CAD build for the part. Positions are in the model's coordinates, mm. Face numbers are marked on the shaded views. A direction names the side the tool comes from. Give positions to 0.01 mm unless a question says otherwise; leave off trailing zeros. Loops run counter-clockwise (first coordinate to the right, second up) from the corner with the lowest first, then second, coordinate; pieces in that order, holes last. Notation, with made-up numbers: M -35.5,-12 L 5.5,-12 A15 cw 5.5,2 Z; hole C -2.5,-30 d3. An arc over 180 degrees is marked long. Answer as CSV lines item,"result".
from build123d import *

# Parameters (mm, degrees)
SKETCH1_W           = 10.5
SKETCH1_H           = 14
SKETCH1_R           = 0.75
SKETCH1_R_2         = 2.25
BOSS_EXTRUDE1_DEPTH = 1.3
SKETCH2_W           = 10.5
SKETCH2_H           = 1.5
BOSS_EXTRUDE2_DEPTH = 14
SKETCH3_W           = 1.4
SKETCH3_H           = 3.3
BOSS_EXTRUDE3_DEPTH = 15.3
SKETCH4_W           = 10.5
SKETCH4_H           = 0.5
BOSS_EXTRUDE4_DEPTH = 1.3
SKETCH5_W           = 10.5
SKETCH5_H           = 1.5
BOSS_EXTRUDE5_DEPTH = 10
SKETCH6_W           = 1
SKETCH6_H           = 13
BOSS_EXTRUDE6_DEPTH = 3
CHAMFER1_SIZE       = 1


with BuildPart() as part:
    # Sketch1 → Boss-Extrude1 (new body)
    with BuildSketch(Plane(origin=(0, 0, 0), x_dir=(1, 0, 0), z_dir=(0, 1, 0))):
        Rectangle(SKETCH1_W, SKETCH1_H)
        with Locations(Location((-3, 3, 0), (0, 0, 270))):
            Circle(SKETCH1_R, mode=Mode.SUBTRACT)
        with Locations(Location((3, 3, 0), (0, 0, 270))):
            Circle(SKETCH1_R, mode=Mode.SUBTRACT)
        with Locations(Location((-3, -3, 0), (0, 0, 270))):
            Circle(SKETCH1_R, mode=Mode.SUBTRACT)
        with Locations(Location((3, -3, 0), (0, 0, 270))):
            Circle(SKETCH1_R, mode=Mode.SUBTRACT)
        with Locations(Location((0, 0, 0), (0, 0, 270))):
            Circle(SKETCH1_R_2, mode=Mode.SUBTRACT)
    extrude(amount=BOSS_EXTRUDE1_DEPTH)

    # Sketch2 → Boss-Extrude2 (add)
    with BuildSketch(Plane(origin=(0, 1.3, 0), x_dir=(1, 0, 0), z_dir=(0, 1, 0))):
        with Locations((0, -6.25)):
            Rectangle(SKETCH2_W, SKETCH2_H)
    extrude(amount=BOSS_EXTRUDE2_DEPTH)

    # Sketch3 → Boss-Extrude3 (add)
    with BuildSketch(Plane.XZ):
        with Locations((-4.55, 8.65)):
            Rectangle(SKETCH3_W, SKETCH3_H)
        with Locations((4.55, 8.65)):
            Rectangle(SKETCH3_W, SKETCH3_H)
    extrude(amount=-BOSS_EXTRUDE3_DEPTH)

    # Sketch4 → Boss-Extrude4 (add)
    with BuildSketch(Plane.XZ):
        with Locations((0, -7.25)):
            Rectangle(SKETCH4_W, SKETCH4_H)
    extrude(amount=-BOSS_EXTRUDE4_DEPTH)

    # Sketch5 → Boss-Extrude5 (add)
    with BuildSketch(Plane.XZ):
        with Locations((0, -8.25)):
            Rectangle(SKETCH5_W, SKETCH5_H)
    extrude(amount=-BOSS_EXTRUDE5_DEPTH)

    # Sketch6 → Boss-Extrude6 (add)
    with BuildSketch(Plane(origin=(0, 1.3, 0), x_dir=(1, 0, 0), z_dir=(0, 1, 0))):
        with Locations((4.75, 1)):
            Rectangle(SKETCH6_W, SKETCH6_H)
        with Locations((-4.75, 1)):
            Rectangle(SKETCH6_W, SKETCH6_H)
    extrude(amount=BOSS_EXTRUDE6_DEPTH)

    # Chamfer1
    chamfer1_edges = [part.edges().sort_by_distance(p)[0] for p in [
        (0, 1.3, -7.5),
    ]]
    chamfer(chamfer1_edges, length=CHAMFER1_SIZE)


solid = part.part
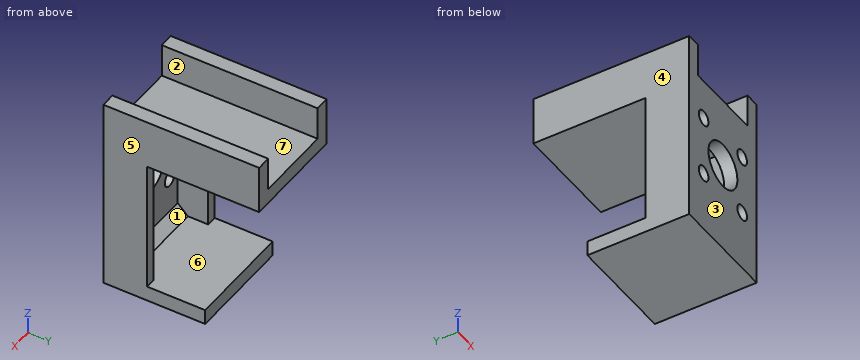
1) Band-saw the part on B-B on z = -3. Give the cut face in (x, y), and give its area (4 significant figures).
Answer below:
outline,"M -5.25,0 L -3.75,0 L -3.75,1.3 L -4.25,1.3 L -4.25,4.3 L -5.25,4.3 Z; M -2.25,0 L 2.25,0 L 2.25,1.3 L -2.25,1.3 Z; M 3.75,0 L 5.25,0 L 5.25,4.3 L 4.25,4.3 L 4.25,1.3 L 3.75,1.3 Z"
area,"15.75 mm^2"
2) Flat gauge pins, fed straight in: pin 1 (4 mm diameter, centred on x = 0.5, z = 2.5, fed in from +Y); pin 2 (1.4 mm diameter, centred on x = -3, z = 3, fed in from -Y); pin 3 (0.5 mm diameter, centred on x = -4.5, z = 1, fed in from +Y). Where does each tip first touch, or does it go through?
Answer below:
pin 1,"stops at y = 1.3"
pin 2,"passes through"
pin 3,"stops at y = 4.3"
3) Mould opens along X. For the marked faces 4, 5, 6 and 7 say: +X half, -X half, draft (parallel to the pull), parting line (faces both ways), or undercut.
Answer below:
face 4,"-X half"
face 5,"+X half"
face 6,"undercut"
face 7,"undercut"
4) Band-saw the part on C-C on y = 1.75. Give the cut face in (x, z), and give its area (3 significant figures).
Answer below:
outline,"M -5.25,-9 L 5.25,-9 L 5.25,10.3 L 3.85,10.3 L 3.85,7 L -3.85,7 L -3.85,10.3 L -5.25,10.3 Z; hole M -4.25,-6.95 L 4.25,-6.95 L 4.25,5.5 L -4.25,5.5 Z"
area,"71.4 mm^2"
5) Band-saw the part on D-D on z = 0. Give the cut face in (x, y), and give its area (3 significant figures).
Answer below:
outline,"M -5.25,0 L -2.25,0 L -2.25,1.3 L -4.25,1.3 L -4.25,4.3 L -5.25,4.3 Z; M 2.25,0 L 5.25,0 L 5.25,4.3 L 4.25,4.3 L 4.25,1.3 L 2.25,1.3 Z"
area,"13.8 mm^2"
6) Which spindle directions (+Z, -Z, +X, -X, +Y, -Y) get a long thin tool onto all of the face, cutting with end or side? Do the marked faces 1, 2 and 3. Say none if no direction does.
Answer below:
face 1,"+Y"
face 2,"+Z, +Y, -Y"
face 3,"+Z, -Z, +X, -X, -Y"
7) Band-saw the part on A-A on x = 3. Give the cut face in (y, z).
Answer below:
outline,"M 0,-9 L 10,-9 L 10,-7.5 L 2.3,-7.5 L 1.3,-6.5 L 1.3,-3.75 L 0,-3.75 Z; M 0,-2.25 L 1.3,-2.25 L 1.3,2.25 L 0,2.25 Z; M 0,3.75 L 1.3,3.75 L 1.3,5.5 L 15.3,5.5 L 15.3,7 L 0,7 Z"
8) Drill centre lines: line 1 (X direction, y = 0.4, z = 3); line 2 (X direction, y = 5, z = 7.75); line 3 (Z direction, x = -3.75, y = 9.5). Where is each one in solid material? Low to high. Write a range as from..to.
Answer below:
line 1,"x = -5.25..-3.75, -2.25..2.25, 3.75..5.25"
line 2,"x = -5.25..-3.85, 3.85..5.25"
line 3,"z = -9..-7.5, 5.5..7"
